Geometry check sheet. Reference: drawing and pictorial views, mm from the part's lowest x, y, z. Round coordinates to 2 decimals unless told otherwise and drop trailing zeros. Write each loop counter-clockwise with the first axis right and the second up, starting at its lowest first coordinate (ties: lowest second). Pieces come first, ordered by that corner, then holes. Notation, with made-up numbers: M -25.5,75.5 L -20.5,75.5 A14 ccw -20.5,83.5 Z; hole C 72.25,63.5 d11. An arc over 180 degrees is marked long. Answer in a Markdown table with one row per item. Add a question column.
1. Sectioned sample at B-B on y = 5.25. Record the cut outline in (x, z), plus the area to 3 significant figures.
2. Go/stop test with flat-tipped pins: pin 1 Ø5 at (x, y) = (20.5, 5.5) entering from -Z; pin 2 Ø3 at (y, z) = (5, 102.5) entering from +X; pin 3 Ø10 at (x, z) = (121, 108) entering from -Y. Record where each tip stops, or that it passes through.
3. Sectioned sample at C-C on x = 34.25. Record the cut outline in (y, z), plus the area to 3 significant figures.
4. Sectioned sample at A-A on z = 117.25. Record the cut outline in (x, y).
5. Sectioned sample at D-D on z = 33.5. Record the cut outline in (x, y), plus the area to 3 significant figures.
6. Material ranges on probe 1 along Z at (x, y) = (101.25, 11.55); probe 2 along X at (y, z) = (11.3, 117.25); probe 3 along Z at (x, y) = (125, 1), recorded low to high.
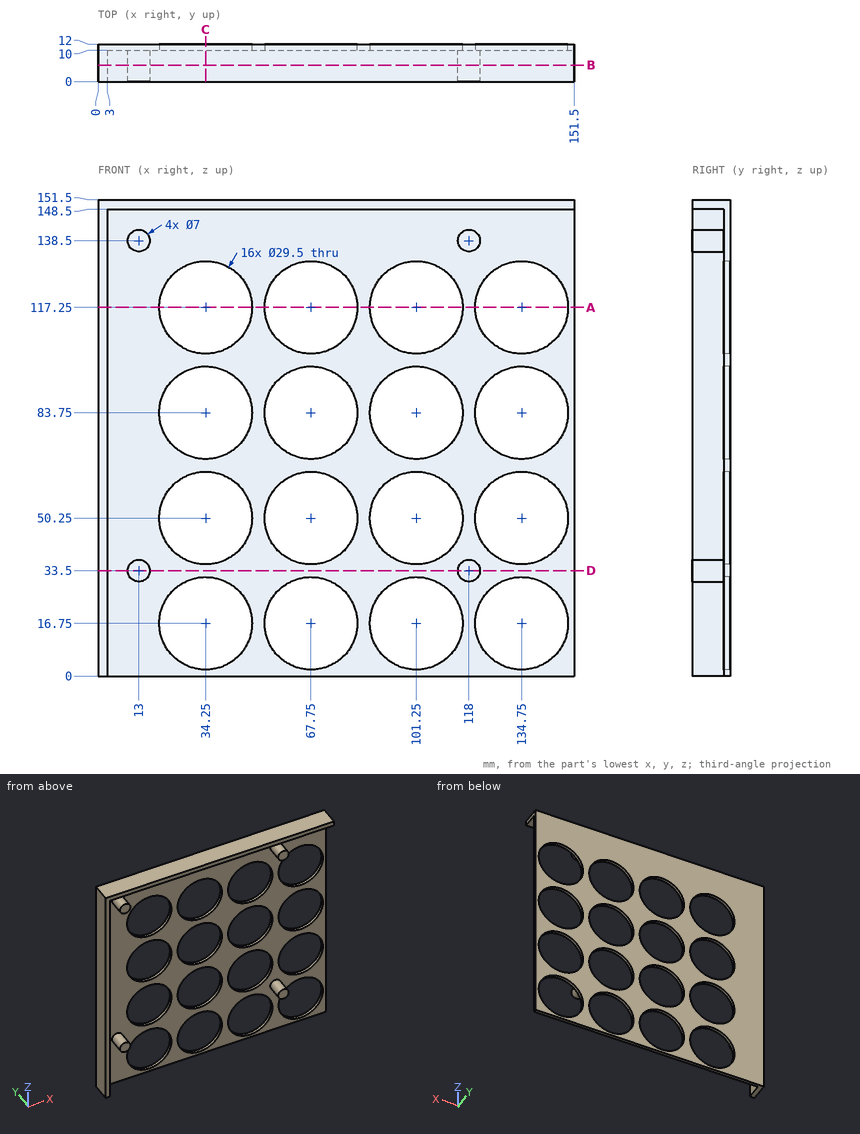
Geometry check:
| question | item | result |
|---|---|---|
| 1 | outline | M 0,0 L 3,0 L 3,148.5 L 151.5,148.5 L 151.5,151.5 L 0,151.5 Z; C 13,33.5 d7; C 13,138.5 d7; C 118,33.5 d7; C 118,138.5 d7 |
| 1 | area | 1,050 mm2 |
| 2 | pin 1 | stops at z = 148.5 |
| 2 | pin 2 | stops at x = 3 |
| 2 | pin 3 | stops at y = 10 |
| 3 | outline | M 0,148.5 L 10,148.5 L 10,132 L 12,132 L 12,151.5 L 0,151.5 Z; M 10,0 L 12,0 L 12,2 L 10,2 Z; M 10,31.5 L 12,31.5 L 12,35.5 L 10,35.5 Z; M 10,65 L 12,65 L 12,69 L 10,69 Z; M 10,98.5 L 12,98.5 L 12,102.5 L 10,102.5 Z |
| 3 | area | 97.0 mm2 |
| 4 | outline | M 0,0 L 3,0 L 3,10 L 19.5,10 L 19.5,12 L 0,12 Z; M 49,10 L 53,10 L 53,12 L 49,12 Z; M 82.5,10 L 86.5,10 L 86.5,12 L 82.5,12 Z; M 116,10 L 120,10 L 120,12 L 116,12 Z; M 149.5,10 L 151.5,10 L 151.5,12 L 149.5,12 Z |
| 5 | outline | M 0,0 L 3,0 L 3,10 L 9.5,10 L 9.5,0 L 16.5,0 L 16.5,10 L 114.5,10 L 114.5,0 L 121.5,0 L 121.5,10 L 151.5,10 L 151.5,12 L 0,12 Z |
| 5 | area | 473 mm2 |
| 6 | probe 1 | z = 0 to 2, 31.5 to 35.5, 65 to 69, 98.5 to 102.5, 132 to 151.5 |
| 6 | probe 2 | x = 0 to 19.5, 49 to 53, 82.5 to 86.5, 116 to 120, 149.5 to 151.5 |
| 6 | probe 3 | z = 148.5 to 151.5 |
